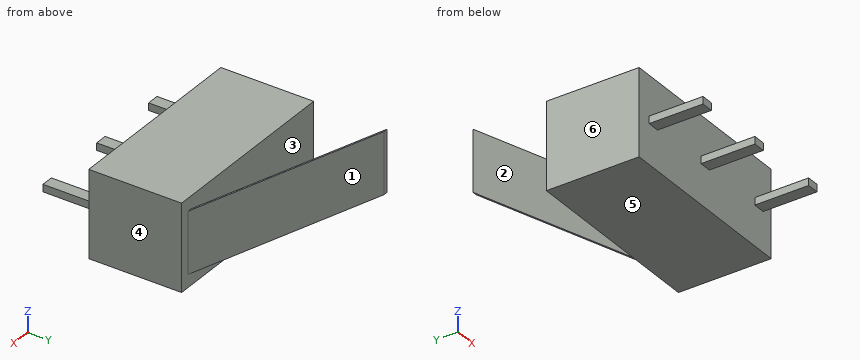
from build123d import *

# Parameters (mm, degrees)
SKETCH1_W           = 12.83
SKETCH1_H           = 5.8
BOSS_EXTRUDE1_DEPTH = 6.2
SKETCH2_W           = 0.31
SKETCH2_H           = 4.1
SKETCH4_W           = 0.81
SKETCH4_H           = 0.49
BOSS_EXTRUDE2_DEPTH = 3.6


with BuildPart() as part:
    # Sketch1 → Boss-Extrude1 (new body)
    with BuildSketch(Plane(origin=(0, 0, 0), x_dir=(1, 0, 0), z_dir=(0, 1, 0))):
        Rectangle(SKETCH1_W, SKETCH1_H)
    extrude(amount=BOSS_EXTRUDE1_DEPTH)

    # Sweep1: sweep along a path in Sketch3
    with BuildLine(Plane.XY.offset(2.9)) as sweep1_path:
        Line((5.621209299, 6.2), (-7.284880173, 10.392583278))
    # Sketch2 → Sweep1 (sweep)
    with BuildSketch(Plane(origin=(0, 6.2, 0), x_dir=(1, 0, 0), z_dir=(0, 1, 0))):
        with Locations((5.621209299, 0)):
            Rectangle(SKETCH2_W, SKETCH2_H)
    sweep(path=sweep1_path.line)

    # Sketch4 → Boss-Extrude2 (add)
    with BuildSketch(Plane.XZ):
        with Locations((-5.04, 0)):
            Rectangle(SKETCH4_W, SKETCH4_H)
        Rectangle(SKETCH4_W, SKETCH4_H)
        with Locations((5.220937528, 0)):
            Rectangle(SKETCH4_W, SKETCH4_H)
    extrude(amount=BOSS_EXTRUDE2_DEPTH)


solid = part.part
Can you work these out from the model? Positions are in its coordinate system, mm. Face numbers are marked on the shaded views. A direction names the side the tool comes from. Give positions to 0.01 mm unless a question says otherwise; leave off trailing zeros. Order: outer loops, then holes, each group sorted by start corner. A loop starts at its lowest first (then second) coordinate and runs counter-clockwise, first axis right, second up. Notation, with made-up numbers: M -0.75,-4.5 L 18.25,-4.5 A30 cw 18.25,21.5 Z; hole C 76.5,10.25 d4. An arc over 180 degrees is marked long. Use a Markdown table: item, result. Add a question column.
Item 1: If I drill on L1, parallel to Y at x = 0, z = -2.55; L2, parallel to X at y = 5, z = 1.9 (3 decimals), over which ranges is the centre line in solid material (lowest first)? Write a range as [from, to].
Item 2: Suppose I cut it at A-A (y = -2.5). List the corners of the cut face in (x, z) for me (3 decimals).
Item 3: Suppose I cut it at C-C (z = -1.3). List the corners of the cut face in (x, y) for me (3 decimals), then the cut area to 3 significant figures.
Item 4: We'd pull the mould along Y, two halves only. Please class the marked faces 1, 2, 3 and 4: +Y half, -Y half, draft (parallel to the pull), parting line (faces both ways), or undercut.
Item 5: Will these pins go through, and if not, where does the flat tip stop? pin 1 (3 mm diameter, centred on y = 7.5, z = 1, fed in from -X) (3 decimals); pin 2 (0.9 mm diameter, centred on x = 5, y = -1.5, fed in from +Z) (3 decimals); pin 3 (1.7 mm diameter, centred on x = 0.5, z = -1.5, fed in from -Y); pin 4 (2 mm diameter, centred on x = 0, y = 9.5, fed in from -Z).
Item 6: For the marked faces 5 and 6, which set-ups out of +Z, -Z, +X, -X, +Y, -Y let a thin tool reach every point of the face, with its end or its side?
Item 7: Suppose I cut it at B-B (x = -5.25). List the corners of the cut face in (y, z) for me (3 decimals), then the cut area to 3 significant figures.
Item 8: Suppose I cut it at D-D (x = -3). List the corners of the cut face in (y, z) for me, then the cut area to 3 significant figures.
Answer sheet:
| question | item | result |
|---|---|---|
| 1 | L1 | y = [0, 6.2] |
| 1 | L2 | x = [-6.415, 6.415] |
| 2 | outline | M -5.445,-0.245 L -4.635,-0.245 L -4.635,0.245 L -5.445,0.245 Z; M -0.405,-0.245 L 0.405,-0.245 L 0.405,0.245 L -0.405,0.245 Z; M 4.816,-0.245 L 5.626,-0.245 L 5.626,0.245 L 4.816,0.245 Z |
| 3 | outline | M -7.44,10.393 L 5.466,6.2 L -6.415,6.2 L -6.415,0 L 6.415,0 L 6.415,6.2 L 5.776,6.2 L -7.13,10.393 Z |
| 3 | area | 80.8 mm² |
| 4 | face 1 | +Y half |
| 4 | face 2 | undercut |
| 4 | face 3 | undercut |
| 4 | face 4 | draft |
| 5 | pin 1 | stops at x = -6.415 |
| 5 | pin 2 | stops at z = 0.245 |
| 5 | pin 3 | stops at y = 0 |
| 5 | pin 4 | passes through |
| 6 | face 5 | -Z, +X, -X, +Y, -Y |
| 6 | face 6 | +Z, -Z, -X, -Y |
| 7 | outline | M -3.6,-0.245 L 0,-0.245 L 0,-2.9 L 6.2,-2.9 L 6.2,2.9 L 0,2.9 L 0,0.245 L -3.6,0.245 Z; M 9.681,-2.05 L 9.782,-2.05 L 9.782,2.05 L 9.681,2.05 Z |
| 7 | area | 38.1 mm² |
| 8 | outline | M 0,-2.9 L 6.2,-2.9 L 6.2,2.9 L 0,2.9 Z; M 8.95,-2.05 L 9.05,-2.05 L 9.05,2.05 L 8.95,2.05 Z |
| 8 | area | 36.4 mm² |
